```python
from build123d import *

# Parameters (mm, degrees)
F0_R     = 3.4
F1_DEPTH = 3.1
F2_R     = 6.3
F3_DEPTH = 3
F4_SIZE  = 2
F5_R     = 4.25
F6_DEPTH = 2.5


with BuildPart() as f1:
    # F0 (on Top) → F1 (new body)
    with BuildSketch(Plane.XY):
        Circle(F0_R)
    extrude(amount=F1_DEPTH)

    # F2 (on face) → F3 (join)
    with BuildSketch(Plane.XY.offset(3.1)):
        Circle(F2_R)
    extrude(amount=F3_DEPTH)

    # F4
    f4_edges = [f1.edges().sort_by_distance(p)[0] for p in [
        (-6.3, 0, 6.1),
    ]]
    chamfer(f4_edges, length=F4_SIZE)

    # F5 (on face) → F6 (cut)
    with BuildSketch(Plane.XY.offset(6.1)):
        Circle(F5_R)
    extrude(amount=-F6_DEPTH, mode=Mode.SUBTRACT)


solid = f1.part
```
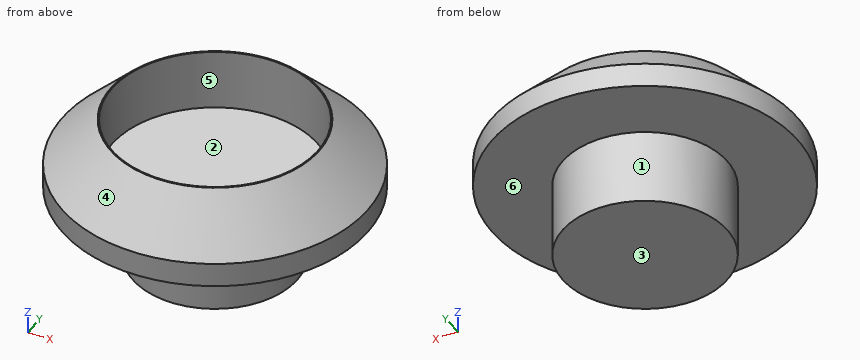
Geometry check sheet. Reference: the model listing, model coordinates, mm. Face numbers are marked on the shaded views. A direction names the side the tool comes from. Coordinates: 2 decimals unless noted, no trailing zeros. Loops run counter-clockwise (first coordinate to the right, second up) from the corner with the lowest first, then second, coordinate; pieces in that order, holes last. Notation, with made-up numbers: (3, 11.5) - (38, 11.5) arc R27 cw to (38, 30.5) - close; hole circle Ø4 at (78, 88). An arc over 180 degrees is marked (long way). One line per item, written item: value. Start each with the question number.
(1) Cross-section at A-A on y = 0. Enter the section's corners in (x, z), plus the area to 3 significant figures.
(2) Tool access check on the marked faces 1, 2 and 3. Record the directions out of +Z, -Z, +X, -X, +Y, -Y that give a thin tool (end or side, any length) a straight path to the whole face; none if there is none.
(3) Mould release check, pull along X, two halves, no side actions. Record for the marked faces 4, 5 and 6: released by +X, released by -X, zero draft, split by the parting line, or undercut.
(4) Cross-section at C-C on z = 2.25. Enter the section's corners in (x, y), plus the area to 3 significant figures.
(5) Material ranges on line 1 (Z direction, x = 3, y = -0.5); line 2 (Z direction, x = -5, y = -3.5); line 3 (Y direction, x = 0, z = 4.45), recorded low to high. Write a range as [from, to].
Results below:
1. outline: (-6.3, 3.1) - (-3.4, 3.1) - (-3.4, 0) - (3.4, 0) - (3.4, 3.1) - (6.3, 3.1) - (6.3, 4.1) - (4.3, 6.1) - (4.25, 6.1) - (4.25, 3.6) - (-4.25, 3.6) - (-4.25, 6.1) - (-4.3, 6.1) - (-6.3, 4.1) - close
1. area: 33.6 mm2
2. face 1: -Z
2. face 2: +Z
2. face 3: -Z, +X, -X, +Y, -Y
3. face 4: split by the parting line
3. face 5: undercut
3. face 6: zero draft
4. outline: circle Ø6.8 at (0, 0)
4. area: 36.3 mm2
5. line 1: z = [0, 3.6]
5. line 2: z = [3.1, 4.3]
5. line 3: y = [-5.95, -4.25], [4.25, 5.95]
